Source: CAD feature listing. Evaluate the final solid. Frame: model axes, mm. A direction names the side the tool comes from. Give positions to 0.01 mm unless a question says otherwise; leave off trailing zeros. Order: outer loops, then holes, each group sorted by start corner. A loop starts at its lowest first (then second) coordinate and runs counter-clockwise, first axis right, second up. Notation, with made-up numbers: M 25.5,-35.5 L 72.5,-35.5 A9 cw 72.5,-18.5 Z; hole C -0.5,-22 d7. An arc over 180 degrees is marked long. Use CSV: the item, a comma, the result in double quotes. Start each with the question number.
Item 1: Section query B-B on z = 21. Count the separate pieces of the cut face and the enclosed holes in it, and give its area (3 significant figures).
Item 2: Section query A-A on x = 0. Return loops of the section in (y, z), and give its area (3 significant figures).
Item 3: Section query C-C on y = 52.5. Return loops of the section in (x, z), and give its area (3 significant figures).
Item 4: First-contact query: pin 1 (10 mm diameter, centred on x = 302, z = -15.5, fed in from +Y); pin 2 (6 mm diameter, centred on x = 214.39, y = -6.95, fed in from -Z); pin 3 (2 mm diameter, centred on x = 255.5, z = 9.5, fed in from -Y); pin 4 (24 mm diameter, centred on x = 164.5, y = -6, fed in from +Z). Flat tips, straight axial feed; report the tip coordinate or a pass-through.
Item 5: Section query D-D on x = 165.5. Return loops of the section in (y, z), and give its area (3 significant figures).
Item 6: Pull-direction query (Y, two-part tool) for faces 4 (the face through (179.64, -3.46, 27.54)), 5 (the face through (271, -17, 15)), 6 (the face through (74.5, 47, 0.2)); classes: +Y half, -Y half, draft (parallel to the pull), parting line (faces both ways), or undercut.
Item 7: Access query for faces 1 (the face through (100, 0, 15)), 2 (the face through (241.768, 21.026, 0.42)), 3 (the face through (34.776, -23.221, -9.93)). Directions: +Z, -Z, +X, -X, +Y, -Y. A direction counts if a zero-diameter tool reaches every point of the face in a straight line with its end or side. Return the directions, or none.
Item 8: Ray query, probe 1 along X at (y, z) = (6, -18.5); probe 2 along X at (y, z) = (-7.5, -22.5); probe 3 along X at (y, z) = (-51, 18). Return the intervals inside material, ascending. Write a range as from..to.
from build123d import *
from build123d.topology import SkipClean

# Parameters (mm, degrees)
LEFT_ARM_DEPTH                = 15
SKETCH2_R                     = 27.5
LEFT_BOSS_DEPTH               = 27.5
LEFT_HEX_DEPTH                = 261.672208
LEFT_HEX_DEPTH_BACK           = 261.672208
SKETCH3_R                     = 70
CENTRE_BOSS_DEPTH             = 30
SKETCH5_W                     = 30
SKETCH5_H                     = 40
RIGHT_ARM_DEPTH               = 175
SKETCH7_R                     = 50
RIGHT_BOSS_DEPTH              = 27.5
SKETCH8_R                     = 30
RIGHT_BOSS_HOLE_DEPTH         = 410.449269
SKETCH9_R                     = 40
CENTRE_HOLE_DEPTH             = 410.807825
SKETCH10_R                    = 27.5
CENTRE_BLOB_DEPTH             = 30
CENTRE_BEAM_REACH             = 240.323
SKETCH11_W                    = 50
SKETCH11_H                    = 30
CENTRE_BEAM_DIRECTION_2_REACH = 240.323
SKETCH12_R                    = 20
CUT_EXTRUDE4_DEPTH            = 5
F_1_4_20_TAPPED_HOLE1_D       = 5.1054
CIRPATTERN1_COUNT             = 8
CUT_OUT_DEPTH                 = 10
FILLET1_R                     = 10
FILLET1_OF_MIRROR2_R          = 10


with BuildPart() as part:
    # Sketch1 → LEFT_ARM (new, symmetric)
    with BuildSketch(Plane.XY):
        with BuildLine():
            Line((-6.678571, 26.676707), (158, 67.904344))
            ThreePointArc((158, 67.904344), (245, 0), (158, -67.904344))
            Line((158, -67.904344), (-6.678571, -26.676707))
            ThreePointArc((-6.678571, -26.676707), (-27.5, 0), (-6.678571, 26.676707))
        make_face()
    extrude(amount=LEFT_ARM_DEPTH, both=True)

    # Sketch2 → LEFT_Boss (add, symmetric)
    with SkipClean():  # the faces are left unmerged after this step: merging them gives an invalid solid
        with BuildSketch(Plane.XY):
            Circle(SKETCH2_R)
        extrude(amount=LEFT_BOSS_DEPTH, both=True)

    # Sketch4 → LEFT_Hex (cut, two sides: drawn at the far end of the back side and taken through both)
    with SkipClean():  # the faces are left unmerged after this step: merging them gives an invalid solid
        with BuildSketch(Plane.XY.offset(27.5).offset(-LEFT_HEX_DEPTH_BACK)):
            Polygon((17.320508, 0), (8.660254, 15), (-8.660254, 15), (-17.320508, 0), (-8.660254, -15), (8.660254, -15), align=None)
        extrude(amount=LEFT_HEX_DEPTH + LEFT_HEX_DEPTH_BACK, mode=Mode.SUBTRACT)

    # Sketch3 → CENTRE_Boss (add, symmetric)
    with BuildSketch(Plane.XY):
        with Locations((175, 0)):
            Circle(SKETCH3_R)
    extrude(amount=CENTRE_BOSS_DEPTH, both=True)

    # Sketch5 → RIGHT_ARM (add)
    with BuildSketch(Plane(origin=(169.723104, -29.926763, 0), x_dir=(0, 0, -1), z_dir=(0.984807753012208, -0.17364817766693072, 0))):
        with Locations((0, 30.388431)):
            Rectangle(SKETCH5_W, SKETCH5_H)
    extrude(amount=RIGHT_ARM_DEPTH)

    # Sketch7 → RIGHT_Boss (add, symmetric)
    with BuildSketch(Plane.XY):
        with Locations((347.341357, -30.388431)):
            Circle(SKETCH7_R)
    extrude(amount=RIGHT_BOSS_DEPTH, both=True)

    # Sketch8 → RIGHT_Boss_Hole (cut, through all)
    with BuildSketch(Plane.XY.offset(27.5)):
        with Locations((347.341357, -30.388431)):
            Circle(SKETCH8_R)
    extrude(amount=-RIGHT_BOSS_HOLE_DEPTH, mode=Mode.SUBTRACT)

    # Sketch9 → CENTRE_Hole (cut, through all)
    with BuildSketch(Plane.XY.offset(30)):
        with Locations((175, 0)):
            Circle(SKETCH9_R)
    extrude(amount=-CENTRE_HOLE_DEPTH, mode=Mode.SUBTRACT)

    # Sketch10 → CENTRE_Blob (add, symmetric)
    with BuildSketch(Plane.XY):
        with Locations((199.620194, -4.341204)):
            Circle(SKETCH10_R)
    extrude(amount=CENTRE_BLOB_DEPTH, both=True)

    # Sketch11 → CENTRE_Beam (add, up to next)
    with BuildSketch(Plane(origin=(175, 0, 0), x_dir=(0, 0, -1), z_dir=(1, 0, 0)), mode=Mode.PRIVATE) as centre_beam_sk1:
        Rectangle(SKETCH11_W, SKETCH11_H)
    centre_beam_tool1 = extrude(centre_beam_sk1.sketch, amount=CENTRE_BEAM_REACH, mode=Mode.PRIVATE) - part.part
    add(centre_beam_tool1.solids().sort_by_distance((175, 0, 0))[0])

    # Sketch11 → CENTRE_Beam direction 2 (add, up to next)
    with BuildSketch(Plane(origin=(175, 0, 0), x_dir=(0, 0, -1), z_dir=(1, 0, 0)), mode=Mode.PRIVATE) as centre_beam_direction_2_sk1:
        Rectangle(SKETCH11_W, SKETCH11_H)
    centre_beam_direction_2_tool1 = extrude(centre_beam_direction_2_sk1.sketch, amount=-CENTRE_BEAM_DIRECTION_2_REACH, mode=Mode.PRIVATE) - part.part
    add(centre_beam_direction_2_tool1.solids().sort_by_distance((175, 0, 0))[0])

    # Sketch12 → Cut-Extrude4 (cut)
    with BuildSketch(Plane.XY.offset(30)):
        with Locations((199.620194, -4.341204)):
            Circle(SKETCH12_R)
    cut_extrude4 = extrude(amount=-CUT_EXTRUDE4_DEPTH, mode=Mode.SUBTRACT)

    # 1/4-20 Tapped Hole1 (through all)
    with Locations(Plane.XY.offset(25)):
        with Locations((184.848078, -1.736482)):
            f_1_4_20_tapped_hole1 = Hole(F_1_4_20_TAPPED_HOLE1_D / 2)

    # CirPattern1: 1/4-20 Tapped Hole1 ×8 about axis
    cirpattern1_axis = Axis((199.620194, -4.341204, 0), (0, 0, 1))
    for i in range(1, CIRPATTERN1_COUNT):
        add(f_1_4_20_tapped_hole1.rotate(cirpattern1_axis, i * 360 / CIRPATTERN1_COUNT), mode=Mode.SUBTRACT)

    # Mirror1: Cut-Extrude4 across plane
    add(cut_extrude4.mirror(Plane.XY), mode=Mode.SUBTRACT)

    # Sketch15 → Cut_OUT (cut)
    with BuildSketch(Plane.XY.offset(15)):
        with BuildLine():
            Line((109.097712, 45.352932), (27.923319, 25.030746))
            ThreePointArc((27.923319, 25.030746), (37.5, 0), (27.923319, -25.030746))
            Line((27.923319, -25.030746), (109.097712, -45.352932))
            ThreePointArc((109.097712, -45.352932), (95, 0), (109.097712, 45.352932))
        make_face()
    cut_out = extrude(amount=-CUT_OUT_DEPTH, mode=Mode.SUBTRACT)

    # Fillet1
    fillet1_edges = [part.edges().sort_by_distance(p)[0] for p in [
        (27.923319, -25.030746, 10),
        (27.923319, 25.030746, 10),
        (109.097712, 45.352932, 10),
        (109.097712, -45.352932, 10),
    ]]
    fillet(fillet1_edges, radius=FILLET1_R)

    # Mirror2: Cut_OUT across plane
    with SkipClean():  # the faces are left unmerged after this step: merging them gives an invalid solid
        add(cut_out.mirror(Plane.XY), mode=Mode.SUBTRACT)

    # Fillet1 of Mirror2
    fillet1_of_mirror2_edges = [part.edges().sort_by_distance(p)[0] for p in [
        (27.923319, -25.030746, -10),
        (27.923319, 25.030746, -10),
        (109.097712, 45.352932, -10),
        (109.097712, -45.352932, -10),
    ]]
    fillet(fillet1_of_mirror2_edges, radius=FILLET1_OF_MIRROR2_R)


solid = part.part
Verdict:
1,separate pieces,"3"
1,enclosed holes,"12"
1,area,"19,800 mm2"
2,outline,"M -28.35,-15 L -27.5,-15 L -27.5,-27.5 L -15,-27.5 L -15,27.5 L -27.5,27.5 L -27.5,15 L -28.35,15 Z; M 15,-27.5 L 27.5,-27.5 L 27.5,-15 L 28.35,-15 L 28.35,15 L 27.5,15 L 27.5,27.5 L 15,27.5 Z"
2,area,"1,430 mm2"
3,outline,"M 96.47,-15 L 128.7,-15 L 128.7,-30 L 221.3,-30 L 221.3,30 L 128.7,30 L 128.7,15 L 96.47,15 Z"
3,area,"6,520 mm2"
4,pin 1,"y = -0.85"
4,pin 2,"z = -25"
4,pin 3,"y = -34.68"
4,pin 4,"z = 30"
5,outline,"M -69.35,-30 L -38.86,-30 L -38.86,30 L -69.35,30 Z; M -15,-25 L 15,-25 L 15,25 L -15,25 Z; M 38.86,-30 L 69.35,-30 L 69.35,30 L 38.86,30 Z"
5,area,"5,160 mm2"
6,face 4,"undercut"
6,face 5,"draft"
6,face 6,"+Y half"
7,face 1,"+Z"
7,face 2,"none"
7,face 3,"-Z"
8,probe 1,"-26.84..-13.86, 13.86..26.84, 105.26..189.36, 192.67..210.04, 213.78..244.74, 313.05..381.63"
8,probe 2,"-26.46..-12.99, 12.99..26.46, 105.4..211.9, 216.88..244.6, 302.89..327.95, 366.74..391.79"
8,probe 3,"127.05..222.95, 301.79..325.54, 369.14..392.9"
